```python
from build123d import *

# Parameters (mm, degrees)
SKETCH1_W           = 172.688303012
SKETCH1_H           = 79
SKETCH1_R           = 2.5
BOSS_EXTRUDE1_DEPTH = 5
CUT_EXTRUDE1_REACH  = 81
SKETCH2_W           = 5
SKETCH2_H           = 1.5


with BuildPart() as part:
    # Sketch1 → Boss-Extrude1 (new body)
    with BuildSketch(Plane.XY):
        Rectangle(SKETCH1_W, SKETCH1_H)
        with Locations((3.337204705, -8.386778216)):
            Circle(SKETCH1_R, mode=Mode.SUBTRACT)
    extrude(amount=BOSS_EXTRUDE1_DEPTH)

    # Sketch2 → Cut-Extrude1 (cut, up to next)
    with BuildSketch(Plane(origin=(0, 39.5, 0), x_dir=(1, 0, 0), z_dir=(0, 1, 0)), mode=Mode.PRIVATE) as cut_extrude1_sk1:
        with Locations((83.844151506, -0.75)):
            Rectangle(SKETCH2_W, SKETCH2_H)
    cut_extrude1_tool1 = extrude(cut_extrude1_sk1.sketch, amount=-CUT_EXTRUDE1_REACH, mode=Mode.PRIVATE) & part.part
    add(cut_extrude1_tool1.solids().sort_by_distance((83.844152, 39.5, 0.75))[0], mode=Mode.SUBTRACT)
    # Sketch2 → Cut-Extrude1 (cut, up to next)
    with BuildSketch(Plane(origin=(0, 39.5, 0), x_dir=(1, 0, 0), z_dir=(0, 1, 0)), mode=Mode.PRIVATE) as cut_extrude1_sk2:
        with Locations((50.306490903, -0.75)):
            Rectangle(SKETCH2_W, SKETCH2_H)
    cut_extrude1_tool2 = extrude(cut_extrude1_sk2.sketch, amount=-CUT_EXTRUDE1_REACH, mode=Mode.PRIVATE) & part.part
    add(cut_extrude1_tool2.solids().sort_by_distance((50.306491, 39.5, 0.75))[0], mode=Mode.SUBTRACT)
    # Sketch2 → Cut-Extrude1 (cut, up to next)
    with BuildSketch(Plane(origin=(0, 39.5, 0), x_dir=(1, 0, 0), z_dir=(0, 1, 0)), mode=Mode.PRIVATE) as cut_extrude1_sk3:
        with Locations((16.768830301, -0.75)):
            Rectangle(SKETCH2_W, SKETCH2_H)
    cut_extrude1_tool3 = extrude(cut_extrude1_sk3.sketch, amount=-CUT_EXTRUDE1_REACH, mode=Mode.PRIVATE) & part.part
    add(cut_extrude1_tool3.solids().sort_by_distance((16.76883, 39.5, 0.75))[0], mode=Mode.SUBTRACT)
    # Sketch2 → Cut-Extrude1 (cut, up to next)
    with BuildSketch(Plane(origin=(0, 39.5, 0), x_dir=(1, 0, 0), z_dir=(0, 1, 0)), mode=Mode.PRIVATE) as cut_extrude1_sk4:
        with Locations((-16.768830301, -0.75)):
            Rectangle(SKETCH2_W, SKETCH2_H)
    cut_extrude1_tool4 = extrude(cut_extrude1_sk4.sketch, amount=-CUT_EXTRUDE1_REACH, mode=Mode.PRIVATE) & part.part
    add(cut_extrude1_tool4.solids().sort_by_distance((-16.76883, 39.5, 0.75))[0], mode=Mode.SUBTRACT)
    # Sketch2 → Cut-Extrude1 (cut, up to next)
    with BuildSketch(Plane(origin=(0, 39.5, 0), x_dir=(1, 0, 0), z_dir=(0, 1, 0)), mode=Mode.PRIVATE) as cut_extrude1_sk5:
        with Locations((-50.306490903, -0.75)):
            Rectangle(SKETCH2_W, SKETCH2_H)
    cut_extrude1_tool5 = extrude(cut_extrude1_sk5.sketch, amount=-CUT_EXTRUDE1_REACH, mode=Mode.PRIVATE) & part.part
    add(cut_extrude1_tool5.solids().sort_by_distance((-50.306491, 39.5, 0.75))[0], mode=Mode.SUBTRACT)
    # Sketch2 → Cut-Extrude1 (cut, up to next)
    with BuildSketch(Plane(origin=(0, 39.5, 0), x_dir=(1, 0, 0), z_dir=(0, 1, 0)), mode=Mode.PRIVATE) as cut_extrude1_sk6:
        with Locations((-83.844151506, -0.75)):
            Rectangle(SKETCH2_W, SKETCH2_H)
    cut_extrude1_tool6 = extrude(cut_extrude1_sk6.sketch, amount=-CUT_EXTRUDE1_REACH, mode=Mode.PRIVATE) & part.part
    add(cut_extrude1_tool6.solids().sort_by_distance((-83.844152, 39.5, 0.75))[0], mode=Mode.SUBTRACT)


solid = part.part
```
Here's how the part is built. I have some questions about the finished solid (model axes, mm). A direction names the side the tool comes from. Coordinates: 2 decimals unless noted, no trailing zeros. Order: outer loops, then holes, each group sorted by start corner. A loop starts at its lowest first (then second) coordinate and runs counter-clockwise, first axis right, second up.
1) We'd pull the mould along X, two halves only. Please class faces 1 (the face through (17, 1, 1.5)), 2 (the face through (-86.344, -1, 3)), 3 (the face through (3.01, -5.91, 2.46)), 4 (the face through (-34, 1, 0)): +X half, -X half, draft (parallel to the pull), parting line (faces both ways), or undercut.
2) Imagine slicing it at A-A on y = 16. List the corners of the cut face in (x, z) for me, and give its area (3 significant figures).
3) Which directions (+Z, -Z, +X, -X, +Y, -Y) give clear straight access to the entire face, cutting with the end or side of a thin tool? Please do faces 5 (the face through (84, 1, 1.5)), 6 (the face through (-84, 1, 1.5)), 7 (the face through (-50, 1, 1.5)).
4) Will these pins go through, and if not, where does the flat tip stop? pin 1 (2.5 mm diameter, centred on x = 49.5, y = 15.5, fed in from -Z); pin 2 (1.6 mm diameter, centred on y = -4.5, z = 0.5, fed in from +X).
5) I need wall thicknesses on line 1 (X direction, y = 36, z = 1.25); line 2 (Z direction, x = 17, y = 3); line 3 (X direction, y = -7, z = 4.75). Which ranges of each line are inside material? Lowest first, please.
Response values:
1. face 1: undercut
1. face 2: -X half
1. face 3: undercut
1. face 4: draft
2. outline: (-86.34, 1.5) - (-81.34, 1.5) - (-81.34, 0) - (-52.81, 0) - (-52.81, 1.5) - (-47.81, 1.5) - (-47.81, 0) - (-19.27, 0) - (-19.27, 1.5) - (-14.27, 1.5) - (-14.27, 0) - (14.27, 0) - (14.27, 1.5) - (19.27, 1.5) - (19.27, 0) - (47.81, 0) - (47.81, 1.5) - (52.81, 1.5) - (52.81, 0) - (81.34, 0) - (81.34, 1.5) - (86.34, 1.5) - (86.34, 5) - (-86.34, 5) - close
2. area: 818 mm2
3. face 5: -Z, +X, +Y, -Y
3. face 6: -Z, -X, +Y, -Y
3. face 7: -Z, +Y, -Y
4. pin 1: stops at z = 1.5
4. pin 2: stops at x = 81.34
5. line 1: x = -81.34 to -52.81, -47.81 to -19.27, -14.27 to 14.27, 19.27 to 47.81, 52.81 to 81.34
5. line 2: z = 1.5 to 5
5. line 3: x = -86.34 to 1.26, 5.42 to 86.34
